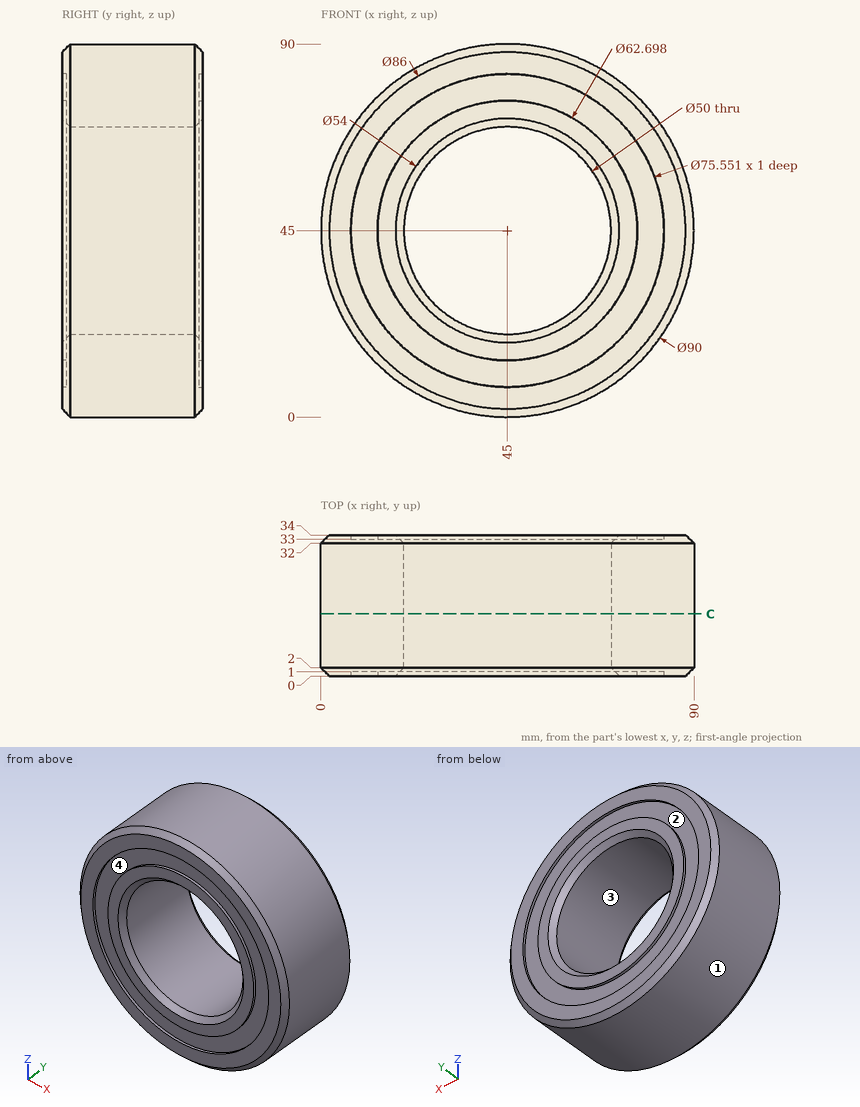
Check sheet for the drawn part. Datum: minimum x, y, z corner. Units: mm. A direction names the side the tool comes from. Round coordinates to 2 decimals unless told otherwise and drop trailing zeros. Loops run counter-clockwise (first coordinate to the right, second up) from the corner with the lowest first, then second, coordinate; pieces in that order, holes last. Notation, with made-up numbers: (71, 40) - (114, 40) arc R24 cw to (114, 62) - close; hole circle Ø9 at (-19.5, -15). An arc over 180 degrees is marked (long way). Write item = value, one per line. Start each with the question number.
1. Set-up check for the marked faces 3 and 4: record each of +Z, -Z, +X, -X, +Y, -Y from which the full face is reachable in a straight line by a thin tool's end or side.
2. Mould release check, pull along Z, two halves, no side actions. Record for the marked faces 1 and 2: released by +Z, released by -Z, zero draft, split by the parting line, or undercut.
3. Thickness scan on line 1 (X direction, y = 28.5, z = 44); line 2 (X direction, y = 32.5, z = 23.5); line 3 (Z direction, x = 26, y = 28). Record the ranges inside material, lowest first.
4. Depth check by flat-ended pin: pin 1 (2 mm diameter, centred on y = 23, z = 70.5, fed in from -X); pin 2 (3 mm diameter, centred on y = 24, z = 75.5, fed in from -X); pin 3 (8 mm diameter, centred on x = 63.5, z = 58, fed in from +Y). Enter the tip coordinate at first touch or a pass-through.
5. Section check C-C on y = 15. Enter the section's corners in (x, z), then the cut area to 3 significant figures.
Working result:
q1.face_3 = +Y, -Y
q1.face_4 = -Y
q2.face_1 = split by the parting line
q2.face_2 = undercut
q3.line_1 = 0.01 to 20.02, 69.98 to 89.99
q3.line_2 = 6.04 to 31.29, 58.71 to 83.96
q3.line_3 = 4.21 to 28.75, 61.25 to 85.79
q4.pin_1 = 7.25
q4.pin_2 = 10.59
q4.pin_3 = 33.61
q5.outline = circle Ø90 at (45, 45); hole circle Ø50 at (45, 45)
q5.area = 4,400 mm^2
